Model file for the job. Use its own axes, mm. Face numbers are marked on the shaded views. A direction names the side the tool comes from. Round coordinates to 2 decimals unless told otherwise and drop trailing zeros. Order: outer loops, then holes, each group sorted by start corner. A loop starts at its lowest first (then second) coordinate and runs counter-clockwise, first axis right, second up. Notation, with made-up numbers: (-20, -6) -> (24, -6) arc R24 cw to (24, 30) -> close; hole circle Ø4 at (38, -39.5). An arc over 180 degrees is marked (long way). Answer as CSV lines item,"result".
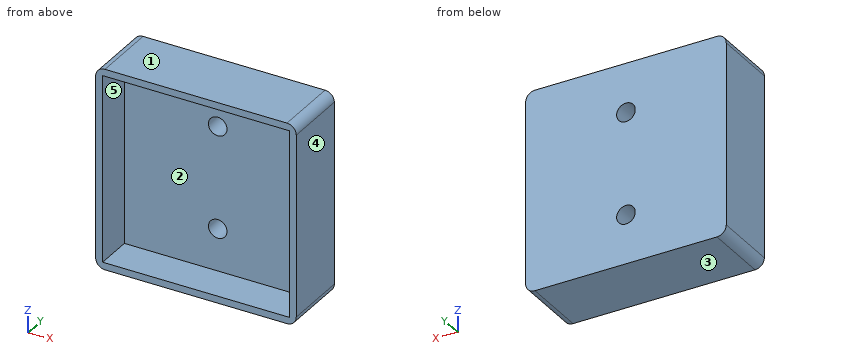
Autodesk Inventor part; units mm, degrees
ref_plane "YZ Plane" through (0, 0, 0) normal (1, 0, 0) x (0, 1, 0)
ref_plane "XZ Plane" through (0, 0, 0) normal (0, 1, 0) x (-1, 0, 0)
ref_plane "XY Plane" through (0, 0, 0) normal (0, 0, 1) x (1, 0, 0)
sketch "Sketch1" plane through (0, 0, 0) normal (0, 1, 0) x (-1, 0, 0)
  line L0 (21.55, 21.55) -> (-21.55, 21.55)
  line L1 (-21.55, 21.55) -> (-21.55, -21.55)
  line L2 (-21.55, -21.55) -> (21.55, -21.55)
  line L3 (21.55, -21.55) -> (21.55, 21.55)
  line L4 (21.55, 21.55) -> (-21.55, -21.55) construction
  line L5 (-21.55, 21.55) -> (21.55, -21.55) construction
  point P0 (0, 0)
  dimension "d0" = 43.1
  dimension "d1" = 43.1
extrude "Extrusion1" add sketch "Sketch1" along normal blind 14
sketch "Sketch2" plane through (0, 0, 0) normal (0, -1, 0) x (1, 0, 0)
  line L0 (-20.05, 20.05) -> (20.05, 20.05)
  line L1 (20.05, 20.05) -> (20.05, -20.05)
  line L2 (20.05, -20.05) -> (-20.05, -20.05)
  line L3 (-20.05, -20.05) -> (-20.05, 20.05)
  line L4 (-20.05, 20.05) -> (20.05, -20.05) construction
  line L5 (20.05, 20.05) -> (-20.05, -20.05) construction
  point P0 (0, 0)
  dimension "d4" = 40.1
  dimension "d5" = 40.1
extrude "Extrusion2" cut sketch "Sketch2" against normal blind 8
fillet "Fillet1" radius 2 4 edges at (-21.55, 7, 21.55) (21.55, 7, 21.55) (21.55, 7, -21.55) (-21.55, 7, -21.55)
sketch "Sketch3" plane through (0, 14, 0) normal (0, 1, 0) x (1, 0, 0)
  line L0 (0, 30.17) -> (0, -30.17)
  circle A0 centre (0, -11) radius 2
  circle A1 centre (0, 11) radius 2
  line L1 (30.17, 0) -> (-30.17, 0)
  point P0 (0, 0)
  dimension "d9" = 4
  dimension "d10" = 22
extrude "Extrusion3" cut sketch "Sketch3" against normal through all
equation "\"d1\" = d0"
equation "\"d5\" = d4"
properties part number "31_Y-Motor_cable_holder"
Q1. Saw through at D-D (x = -8). Write the cut outline in (y, z).
Checks:
outline,"(0, -21.55) -> (14, -21.55) -> (14, 21.55) -> (0, 21.55) -> (0, 20.05) -> (8, 20.05) -> (8, -20.05) -> (0, -20.05) -> close"
Q2. Mould opens along Z. For the marked faces 1, 2 and 3 say: +Z half, -Z half, draft (parallel to the pull), parting line (faces both ways), or undercut.
Checks:
face 1,"+Z half"
face 2,"undercut"
face 3,"-Z half"
Q3. Saw through at C-C (x = 0). Write the cut outline in (y, z), plus the area to 3 significant figures.
Checks:
outline,"(0, -21.55) -> (14, -21.55) -> (14, -13) -> (8, -13) -> (8, -20.05) -> (0, -20.05) -> close; (0, 20.05) -> (8, 20.05) -> (8, 13) -> (14, 13) -> (14, 21.55) -> (0, 21.55) -> close; (8, -9) -> (14, -9) -> (14, 9) -> (8, 9) -> close"
area,"235 mm²"
Q4. Tool access for the marked faces 4 and 5: list every direction of +Z, -Z, +X, -X, +Y, -Y with a clear straight run to the whole face (end or side of a thin tool).
Checks:
face 4,"+Z, -Z, +X, +Y, -Y"
face 5,"-Y"
Q5. Wall check: L1, parallel to Z at x = 0, y = 12.5; L2, parallel to X at y = 10.8, z = -11; L3, parallel to Z at x = 4, y = 2. Give the ranges that are in metal, low to high. Write a range as [from, to].
Checks:
L1,"[-21.55, -13], [-9, 9], [13, 21.55]"
L2,"[-21.55, -2], [2, 21.55]"
L3,"[-21.55, -20.05], [20.05, 21.55]"
Q6. Saw through at B-B (z = 11). Write the cut outline in (x, y).
Checks:
outline,"(-21.55, 0) -> (-20.05, 0) -> (-20.05, 8) -> (-2, 8) -> (-2, 14) -> (-21.55, 14) -> close; (2, 8) -> (20.05, 8) -> (20.05, 0) -> (21.55, 0) -> (21.55, 14) -> (2, 14) -> close"
Q7. Flat gauge pins, fed straight in: pin 1 (2.5 mm diameter, centred on x = 0, z = 11, fed in from -Y) (3 decimals); pin 2 (12 mm diameter, centred on x = -0.5, z = 5, fed in from -Y). Where does each tip first touch, or does it go through?
Checks:
pin 1,"through"
pin 2,"y = 8"
Q8. Saw through at A-A (y = 9.25). Write the cut outline in (x, z), plus the area to 3 significant figures.
Checks:
outline,"(-21.55, -19.55) arc R2 ccw to (-19.55, -21.55) -> (19.55, -21.55) arc R2 ccw to (21.55, -19.55) -> (21.55, 19.55) arc R2 ccw to (19.55, 21.55) -> (-19.55, 21.55) arc R2 ccw to (-21.55, 19.55) -> close; hole circle Ø4 at (0, -11); hole circle Ø4 at (0, 11)"
area,"1,830 mm²"
